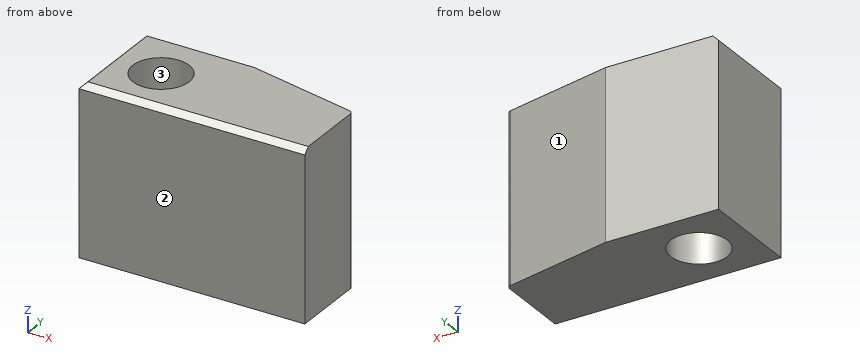
from build123d import *

# Parameters (mm, degrees)
SKETCH1_R           = 2.5
BOSS_EXTRUDE1_DEPTH = 15
FILLET1_R           = 0.4
CHAMFER2_SIZE       = 0.5


with BuildPart() as part:
    # Sketch1 → Boss-Extrude1 (new body)
    with BuildSketch(Plane.XY):
        Polygon((5.5, 4.5), (15.5, 2.374434383), (15.5, -4.5), (-4.5, -4.5), (-4.5, 4.5), align=None)
        Circle(SKETCH1_R, mode=Mode.SUBTRACT)
    extrude(amount=BOSS_EXTRUDE1_DEPTH)

    # Fillet1
    fillet1_edges = [part.edges().sort_by_distance(p)[0] for p in [
        (15.5, 2.374434383, 7.5),
    ]]
    fillet(fillet1_edges, radius=FILLET1_R)

    # Chamfer2
    chamfer2_edges = [part.edges().sort_by_distance(p)[0] for p in [
        (-4.5, 0, 15),
        (5.5, -4.5, 15),
    ]]
    chamfer(chamfer2_edges, length=CHAMFER2_SIZE)


solid = part.part
For this review, take the finished solid that the model builds, in its own axes (mm). Face numbers are marked on the shaded views. Round coordinates to 2 decimals unless told otherwise and drop trailing zeros. Order: outer loops, then holes, each group sorted by start corner. A loop starts at its lowest first (then second) coordinate and runs counter-clockwise, first axis right, second up. Notation, with made-up numbers: M -32,66 L -13,66 A18 cw -13,101 Z; hole C 70,-27.75 d7. An arc over 180 degrees is marked long. Use a Markdown table: item, result. Add a question column.
Item 1: Add section B-B, the plane x = 0. Give the boundary of the cut face in (y, z).
Item 2: Mouldability with a two-part tool opening along X and no side actions: class the marked faces 1, 2 and 3 as released by +X, released by -X, zero draft, split by the parting line, or undercut.
Item 3: Add section C-C, the plane z = 4. Give the boundary of the cut face in (x, y).
Item 4: Add section D-D, the plane y = 3.5. Give the boundary of the cut face in (x, z).
Item 5: To check wall thickness, follow line 1 along Y through (x, z) = (0, 10.25); line 2 along X through (y, z) = (-1.5, 9); line 3 along Y through (x, z) = (-0.5, 12.5). State the ranges of each line that lie inside material, in increasing order.
Item 6: Add section A-A, the plane y = -2. Give the boundary of the cut face in (x, z).
Geometry results:
| question | item | result |
|---|---|---|
| 1 | outline | M -4.5,0 L -2.5,0 L -2.5,15 L -4,15 L -4.5,14.5 Z; M 2.5,0 L 4.5,0 L 4.5,15 L 2.5,15 Z |
| 2 | face 1 | released by +X |
| 2 | face 2 | zero draft |
| 2 | face 3 | undercut |
| 3 | outline | M -4.5,-4.5 L 15.5,-4.5 L 15.5,2.05 A0.4 ccw 15.18,2.44 L 5.5,4.5 L -4.5,4.5 Z; hole C 0,0 d5 |
| 4 | outline | M -4.5,0 L 10.2,0 L 10.2,15 L -4,15 L -4.5,14.5 Z |
| 5 | line 1 | y = -4.5 to -2.5, 2.5 to 4.5 |
| 5 | line 2 | x = -4.5 to -2, 2 to 15.5 |
| 5 | line 3 | y = -4.5 to -2.45, 2.45 to 4.5 |
| 6 | outline | M -4.5,0 L -1.5,0 L -1.5,15 L -4,15 L -4.5,14.5 Z; M 1.5,0 L 15.5,0 L 15.5,15 L 1.5,15 Z |
